from build123d import *

# Parameters (mm, degrees)
SKETCH1_R           = 4.5
BOSS_EXTRUDE1_DEPTH = 3.5
CUT_EXTRUDE1_DEPTH  = 1.5
FILLET1_R           = 0.5
FILLET2_R           = 0.2
CHAMFER1_SIZE       = 0.5


with BuildPart() as part:
    # Sketch1 → Boss-Extrude1 (new body)
    with BuildSketch(Plane.XY):
        with BuildLine():
            ThreePointArc((7.476559852, 17.407502934), (0, 25.5), (-7.476559852, 17.407502934))
            ThreePointArc((-7.476559852, 17.407502934), (-10.093544717, 5.827510759), (-18.813619684, -2.228860702))
            ThreePointArc((-18.813619684, -2.228860702), (-22.083647797, -12.75), (-11.337059831, -15.178642232))
            ThreePointArc((-11.337059831, -15.178642232), (0, -11.655021518), (11.337059831, -15.178642232))
            ThreePointArc((11.337059831, -15.178642232), (22.083647797, -12.75), (18.813619684, -2.228860702))
            ThreePointArc((18.813619684, -2.228860702), (10.093544717, 5.827510759), (7.476559852, 17.407502934))
        make_face()
        with Locations((0, 18)):
            Circle(SKETCH1_R, mode=Mode.SUBTRACT)
        with Locations((15.588457268, -9)):
            Circle(SKETCH1_R, mode=Mode.SUBTRACT)
        with Locations((-15.588457268, -9)):
            Circle(SKETCH1_R, mode=Mode.SUBTRACT)
    extrude(amount=BOSS_EXTRUDE1_DEPTH)

    # Sketch2 → Revolve4 (revolve)
    with BuildSketch(Plane(origin=(0, 0, 0), x_dir=(0, 0, -1), z_dir=(1, 0, 0)), mode=Mode.PRIVATE) as revolve4_sk:
        Polygon((-53.5, 2.5), (-43.5, 2.5), (-43.5, 4), (-42, 4), (-42, 2.5), (-3.5, 2.5), (-3.5, 0), (-53.5, 0), align=None)
    revolve(revolve4_sk.sketch.rotate(Axis((0, 0, 49.596889026), (0, 0, -1)), 90), axis=Axis((0, 0, 49.596889026), (0, 0, -1)))

    # Sketch6 → Cut-Extrude1 (cut)
    with BuildSketch(Plane(origin=(2.5, 0, 0), x_dir=(0, 0, -1), z_dir=(1, 0, 0))):
        with BuildLine():
            Line((-51, 0.75), (-46, 0.75))
            ThreePointArc((-46, 0.75), (-45.25, 0), (-46, -0.75))
            Line((-46, -0.75), (-51, -0.75))
            ThreePointArc((-51, -0.75), (-51.75, 0), (-51, 0.75))
        make_face()
    extrude(amount=-CUT_EXTRUDE1_DEPTH, mode=Mode.SUBTRACT)

    # Fillet1
    fillet1_edges = [part.edges().sort_by_distance(p)[0] for p in [
        (-10.093544717, 5.827510759, 3.5),
        (-22.083647797, -12.75, 3.5),
        (0, -11.655021518, 3.5),
        (22.083647797, -12.75, 3.5),
        (10.093544717, 5.827510759, 3.5),
        (0, 25.5, 3.5),
    ]]
    fillet(fillet1_edges, radius=FILLET1_R)

    # Fillet2
    fillet2_edges = [part.edges().sort_by_distance(p)[0] for p in [
        (-4, 0, 42),
        (-4, 0, 43.5),
    ]]
    fillet(fillet2_edges, radius=FILLET2_R)

    # Chamfer1
    chamfer1_edges = [part.edges().sort_by_distance(p)[0] for p in [
        (-2.5, 0, 53.5),
    ]]
    chamfer(chamfer1_edges, length=CHAMFER1_SIZE)


solid = part.part
The listing builds one solid part. Answer for the finished solid, in the listing's coordinates (mm). A direction names the side the tool comes from. Give positions to 0.01 mm unless a question says otherwise; leave off trailing zeros. Write each loop counter-clockwise with the first axis right and the second up, starting at its lowest first coordinate (ties: lowest second). Pieces come first, ordered by that corner, then holes. Notation, with made-up numbers: (66.25, 85.25) -> (73.25, 85.25) arc R23 cw to (73.25, 121.25) -> close; hole circle Ø5 at (1, 88). An arc over 180 degrees is marked (long way). Use a Markdown table: item, result.
(1) Section C-C, the plane z = 30.5 is taken. Determine the outline of the cut face in (x, y).
Return value:
| item | result |
|---|---|
| outline | circle Ø5 at (0, 0) |
(2) Flat-ended cylindrical pins translate along their axes: P1, Ø7, axis at x = -15.59, y = -9, coming from the -Z side; P2, Ø5, axis at y = -4, z = 32, coming from the -X side; P3, Ø0.7, axis at x = 2, z = 49, coming from the -Y side; P4, Ø12, axis at y = -2.5, z = 14.5, coming from the -X side. Find the tip coordinate at first contact, or state that the pin passes through.
Return value:
| item | result |
|---|---|
| P1 | through |
| P2 | x = -2 |
| P3 | y = -1.88 |
| P4 | x = -2.5 |
(3) Find the intervals of material crossed by probe 1 along Z at (x, y) = (2, -4.5); probe 2 along X at (y, z) = (-1, 51); probe 3 along X at (y, z) = (2, 14), in increasing order. Write a range as from..to.
Return value:
| item | result |
|---|---|
| probe 1 | 0..3.5 |
| probe 2 | -2.29..2.29 |
| probe 3 | -1.5..1.5 |
(4) Section A-A, the plane x = 0 is taken. Determine the outline of the cut face in (y, z), then the cut area to 3 significant figures.
Return value:
| item | result |
|---|---|
| outline | (-11.66, 0) -> (13.5, 0) -> (13.5, 3.5) -> (2.5, 3.5) -> (2.5, 42) -> (3.8, 42) arc R0.2 ccw to (4, 42.2) -> (4, 43.3) arc R0.2 ccw to (3.8, 43.5) -> (2.5, 43.5) -> (2.5, 53) -> (2, 53.5) -> (-2, 53.5) -> (-2.5, 53) -> (-2.5, 43.5) -> (-3.8, 43.5) arc R0.2 ccw to (-4, 43.3) -> (-4, 42.2) arc R0.2 ccw to (-3.8, 42) -> (-2.5, 42) -> (-2.5, 3.5) -> (-11.16, 3.5) arc R0.5 ccw to (-11.66, 3) -> close; (22.5, 0) -> (25.5, 0) -> (25.5, 3) arc R0.5 ccw to (25, 3.5) -> (22.5, 3.5) -> close |
| area | 353 mm2 |
(5) Section B-B, the plane y = -9 is taken. Give the number of separate pieces and of enclosed holes in the cut face, then the cut area to 3 significant figures.
Return value:
| item | result |
|---|---|
| separate pieces | 3 |
| enclosed holes | 0 |
| area | 98.5 mm2 |
(6) For faces 4 (the cylindrical face through (1.76, -0.02, 51.75)), 5 (the cylindrical face through (-0.867, 3.905, 42.742)), 6 (the flat face through (-0.9, 2.5, 42)), determine the directions among +Z, -Z, +X, -X, +Y, -Y from which every point of the face is accessible in a straight line to the end or side of a thin tool.
Return value:
| item | result |
|---|---|
| face 4 | +X |
| face 5 | +Z |
| face 6 | none |
(7) Determine the mould class of faces 1 (the cylindrical face through (1.76, 0.02, 45.25)), 2 (the flat face through (0, 0, 0)), 3 (the cylindrical face through (-2.5, -0.1, 48.2)) for opening direction Y: released by +Y, released by -Y, zero draft, split by the parting line, or undercut.
Return value:
| item | result |
|---|---|
| face 1 | undercut |
| face 2 | zero draft |
| face 3 | split by the parting line |
